from build123d import *

# Parameters (mm, degrees)
F0_W      = 380
F0_H      = 350
F1_DEPTH  = 100
F2_W      = 170
F2_H      = 50
F2_W_2    = 65
F2_H_2    = 160
F3_DEPTH  = 100.001
F4_W      = 50
F4_H      = 70
F4_W_2    = 160
F5_DEPTH  = 380.001
F7_R      = 15
F8_DEPTH  = 25
F9_R      = 15
F10_DEPTH = 25
F11_W     = 160
F11_H     = 60
F12_DEPTH = 25
F13_W     = 160
F13_H     = 60
F14_DEPTH = 25
F15_W     = 160
F15_H     = 160
F16_DEPTH = 25
F17_W     = 210
F17_H     = 210
F18_DEPTH = 40
F19_W     = 100
F19_H     = 150
F20_DEPTH = 25
F21_W     = 160
F21_H     = 25
F22_DEPTH = 350.001
F24_DEPTH = 25


with BuildPart() as f1:
    # F0 (on Top) → F1 (new body)
    with BuildSketch(Plane.XY):
        Rectangle(F0_W, F0_H)
    extrude(amount=F1_DEPTH)

    # F2 (on face) → F3 (cut, through all)
    with BuildSketch(Plane.XY.offset(100)):
        with Locations((0, 130)):
            Rectangle(F2_W, F2_H)
        with Locations((137.5, 130)):
            Rectangle(F2_W_2, F2_H)
        with Locations((137.5, 0)):
            Rectangle(F2_W_2, F2_H_2)
        with Locations((137.5, -130)):
            Rectangle(F2_W_2, F2_H)
        with Locations((0, -130)):
            Rectangle(F2_W, F2_H)
        with Locations((-137.5, -130)):
            Rectangle(F2_W_2, F2_H)
        with Locations((-137.5, 0)):
            Rectangle(F2_W_2, F2_H_2)
        with Locations((-137.5, 130)):
            Rectangle(F2_W_2, F2_H)
    extrude(amount=-F3_DEPTH, mode=Mode.SUBTRACT)

    # F4 (on face) → F5 (cut, through all)
    with BuildSketch(Plane.YZ.offset(190)):
        with Locations((-130, 50)):
            Rectangle(F4_W, F4_H)
        with Locations((0, 50)):
            Rectangle(F4_W_2, F4_H)
        with Locations((130, 50)):
            Rectangle(F4_W, F4_H)
    extrude(amount=-F5_DEPTH, mode=Mode.SUBTRACT)

    # F7 (on face) → F8 (cut)
    with BuildSketch(Plane.XZ.offset(175)):
        with Locations((-150, 25)):
            Circle(F7_R)
        with Locations((150, 25)):
            Circle(F7_R)
    extrude(amount=-F8_DEPTH, mode=Mode.SUBTRACT)

    # F9 (on face) → F10 (cut)
    with BuildSketch(Plane(origin=(0, 175, 0), x_dir=(-1, 0, 0), z_dir=(0, 1, 0))):
        with Locations((-150, 25)):
            Circle(F9_R)
        with Locations((150, 25)):
            Circle(F9_R)
    extrude(amount=-F10_DEPTH, mode=Mode.SUBTRACT)

    # F11 (on face) → F12 (cut)
    with BuildSketch(Plane(origin=(0, 175, 0), x_dir=(-1, 0, 0), z_dir=(0, 1, 0))):
        with Locations((0, 50)):
            Rectangle(F11_W, F11_H)
    extrude(amount=-F12_DEPTH, mode=Mode.SUBTRACT)

    # F13 (on face) → F14 (cut)
    with BuildSketch(Plane.XZ.offset(175)):
        with Locations((0, 50)):
            Rectangle(F13_W, F13_H)
    extrude(amount=-F14_DEPTH, mode=Mode.SUBTRACT)

    # F15 (on face) → F16 (cut)
    with BuildSketch(Plane(origin=(0, 0, 0), x_dir=(1, 0, 0), z_dir=(0, 0, -1))):
        Rectangle(F15_W, F15_H)
    extrude(amount=-F16_DEPTH, mode=Mode.SUBTRACT)

    # F17 (on face) → F18 (join)
    with BuildSketch(Plane(origin=(0, 0, 85), x_dir=(1, 0, 0), z_dir=(0, 0, -1))):
        Rectangle(F17_W, F17_H)
    extrude(amount=F18_DEPTH)

    # F19 (on face) → F20 (cut)
    with BuildSketch(Plane.XY.offset(100)):
        with Locations((-25, 0)):
            Rectangle(F19_W, F19_H)
    extrude(amount=-F20_DEPTH, mode=Mode.SUBTRACT)

    # F21 (on face) → F22 (cut, through all)
    with BuildSketch(Plane(origin=(0, 175, 0), x_dir=(-1, 0, 0), z_dir=(0, 1, 0))):
        with Locations((0, 32.5)):
            Rectangle(F21_W, F21_H)
    extrude(amount=-F22_DEPTH, mode=Mode.SUBTRACT)

    # F23 (on face) → F24 (cut)
    with BuildSketch(Plane.XZ.offset(175)):
        Polygon((-105, 80), (-170, 80), (-170, 60), (-120, 60), (-120, 20), (-105, 20), align=None)
    extrude(amount=-F24_DEPTH, mode=Mode.SUBTRACT)


solid = f1.part
The listing builds one solid part. Answer for the finished solid, in the listing's coordinates (mm). A direction names the side the tool comes from. Coordinates: 2 decimals unless noted, no trailing zeros. Loops run counter-clockwise (first coordinate to the right, second up) from the corner with the lowest first, then second, coordinate; pieces in that order, holes last.
1) Flat-ended cylindrical pins translate along their axes: pin 1 Ø1.5 at (x, z) = (24, 53) entering from -Y; pin 2 Ø16 at (x, y) = (175.5, -139) entering from -Z; pin 3 Ø8 at (y, z) = (-37.5, 45.5) entering from -X. Find the tip coordinate at first contact, or state that the pin passes through.
2) Find section B-B on y = -60. Give the number of separate pieces and of enclosed holes in the cut face, then the cut area to 3 significant figures.
3) Find section A-A on x = 150. Write down the section's boundary in (y, z), then the cut area to 3 significant figures.
4) Find the intervals of material crossed by L1, parallel to Y at x = 166.5, z = 94.5; L2, parallel to Z at x = -150, y = -161.75; L3, parallel to Y at x = -115, z = 49, in increasing order.
5) A tool of negligible diameter and unlimited length cuts with its end or side. For faces 1 (the face through (164.985, 165.14, 25.66)), 2 (the face through (-92, -1, 15)), 3 (the face through (105, 130, 93)), from which of +Z, -Z, +X, -X, +Y, -Y can it reach the whole face along a straight path? Write none if from no direction.
6) Determine the mould class of faces 4 (the face through (-170, -130, 8)), 5 (the face through (-44.9, 80.2, 0)), 6 (the face through (3, 155, 16)) for opening direction Y: pulls with the +Y half, pulls with the -Y half, needs draft (parallel to the pull), parting line crosses it, or undercut.
Values:
1. pin 1: stops at y = -105
1. pin 2: stops at z = 0
1. pin 3: stops at x = -105
2. separate pieces: 7
2. enclosed holes: 0
2. area: 11,000 mm2
3. outline: (-175, 0) - (-155, 0) - (-155, 10) - (-175, 10) - close; (-175, 40) - (-155, 40) - (-155, 100) - (-175, 100) - close; (-105, 0) - (-80, 0) - (-80, 100) - (-105, 100) - close; (80, 0) - (105, 0) - (105, 100) - (80, 100) - close; (155, 0) - (175, 0) - (175, 10) - (155, 10) - close; (155, 40) - (175, 40) - (175, 100) - (155, 100) - close
3. area: 7,800 mm2
4. L1: y = -175 to -155, -105 to -80, 80 to 105, 155 to 175
4. L2: z = 0 to 10, 40 to 60, 80 to 100
4. L3: y = -105 to -80, 80 to 105, 155 to 175
5. face 1: +Y
5. face 2: +X, -X
5. face 3: +Z, -Z
6. face 4: undercut
6. face 5: needs draft
6. face 6: undercut
